```python
from build123d import *

# Parameters (mm, degrees)
ESBO_O1_R                = 6.5
RESSALTO_EXTRUS_O1_DEPTH = 15
ESBO_O4_R                = 4.5
CORTE_EXTRUS_O1_DEPTH    = 3.1
ESBO_O5_R                = 3.25
CORTE_EXTRUS_O2_DEPTH    = 16.036954479
CHANFRO1_SIZE            = 0.5
FILETE1_R                = 0.5
FILETE2_R                = 0.5


with BuildPart() as part:
    # Esboço1 → Ressalto-extrusão1 (new body)
    with BuildSketch(Plane(origin=(0, 0, 0), x_dir=(1, 0, 0), z_dir=(0, 1, 0))):
        with Locations(Location((0, 0, 0), (0, 0, 270))):
            Circle(ESBO_O1_R)
    extrude(amount=RESSALTO_EXTRUS_O1_DEPTH)

    # Esboço4 → Corte-extrusão1 (cut)
    with BuildSketch(Plane.XZ):
        with Locations(Location((0, 0, 0), (0, 0, 270))):
            Circle(ESBO_O4_R)
    extrude(amount=-CORTE_EXTRUS_O1_DEPTH, mode=Mode.SUBTRACT)

    # Esboço5 → Corte-extrusão2 (cut, through all)
    with BuildSketch(Plane.XZ.offset(-3.1)):
        with Locations(Location((0, 0, 0), (0, 0, 270))):
            Circle(ESBO_O5_R)
    extrude(amount=-CORTE_EXTRUS_O2_DEPTH, mode=Mode.SUBTRACT)

    # Chanfro1
    chanfro1_edges = [part.edges().sort_by_distance(p)[0] for p in [
        (0, 0, 4.5),
    ]]
    chamfer(chanfro1_edges, length=CHANFRO1_SIZE)

    # Filete1
    filete1_edges = [part.edges().sort_by_distance(p)[0] for p in [
        (0, 3.1, 3.25),
    ]]
    fillet(filete1_edges, radius=FILETE1_R)

    # Filete2
    filete2_edges = [part.edges().sort_by_distance(p)[0] for p in [
        (0, 15, 3.25),
    ]]
    fillet(filete2_edges, radius=FILETE2_R)


solid = part.part
```
Read the model definition and answer for the solid it produces. Units are mm, in the model's axes. A direction names the side the tool comes from. Round coordinates to 2 decimals unless told otherwise and drop trailing zeros. Write each loop counter-clockwise with the first axis right and the second up, starting at its lowest first coordinate (ties: lowest second). Pieces come first, ordered by that corner, then holes. Notation, with made-up numbers: (10.5, 19) - (57.5, 19) arc R20 ccw to (57.5, 54) - close; hole circle Ø1 at (78, 0). An arc over 180 degrees is marked (long way). One line per item, written item: value.
Q1. Find section A-A (x = 0). Determine the outline of the cut face in (y, z), and give its area (3 significant figures).
The answers:
outline: (0, -6.5) - (15, -6.5) - (15, -3.75) arc R0.5 ccw to (14.5, -3.25) - (3.6, -3.25) arc R0.5 ccw to (3.1, -3.75) - (3.1, -4.5) - (0.5, -4.5) - (0, -5) - close; (0, 5) - (0.5, 4.5) - (3.1, 4.5) - (3.1, 3.75) arc R0.5 ccw to (3.6, 3.25) - (14.5, 3.25) arc R0.5 ccw to (15, 3.75) - (15, 6.5) - (0, 6.5) - close
area: 89.3 mm2
Q2. For a pull along Z with two mould halves and no side action, classify faces 1 (the cylindrical face through (-3.955, 7.395, -5.158)), 2 (the flat face through (-3, 15, 3)), 3 (the flat face through (4, 3.1, 1)) as pulls with the +Z half, pulls with the -Z half, needs draft (parallel to the pull), parting line crosses it, or undercut.
The answers:
face 1: parting line crosses it
face 2: needs draft
face 3: undercut
Q3. Straight lines are drawn through the part: line 1 (X direction, y = 8, z = 0); line 2 (X direction, y = 2, z = 0); line 3 (Z direction, x = 1, y = 13). For each, find the intervals that lie inside material, in ascending order. Write a range as from..to.
The answers:
line 1: x = -6.5..-3.25, 3.25..6.5
line 2: x = -6.5..-4.5, 4.5..6.5
line 3: z = -6.42..-3.09, 3.09..6.42
Q4. Find section B-B (z = 0). Determine the outline of the cut face in (x, y).
The answers:
outline: (-6.5, 0) - (-5, 0) - (-4.5, 0.5) - (-4.5, 3.1) - (-3.75, 3.1) arc R0.5 ccw to (-3.25, 3.6) - (-3.25, 14.5) arc R0.5 ccw to (-3.75, 15) - (-6.5, 15) - close; (3.25, 3.6) arc R0.5 ccw to (3.75, 3.1) - (4.5, 3.1) - (4.5, 0.5) - (5, 0) - (6.5, 0) - (6.5, 15) - (3.75, 15) arc R0.5 ccw to (3.25, 14.5) - close
Q5. Each of these flat-tipped pins is pushed along its axis until it touches: P1, Ø2.5, axis at x = 1, z = 1, coming from the -Y side; P2, Ø3, axis at y = 13.5, z = -4.5, coming from the +X side; P3, Ø1, axis at x = -5, y = 3, coming from the +Z side; P4, Ø1.5, axis at x = 3, y = 3.5, coming from the +Z side. Where does it stop, or does it pass through?
The answers:
P1: passes through
P2: stops at x = 5.77
P3: stops at z = 4.69
P4: stops at z = 6.1
Q6. Which of the six approach directions +Z, -Z, +X, -X, +Y, -Y give full straight-line access (tool end or side, diameter ignored) to faces 4 (the cylindrical face through (-1.978, 8.974, 2.579)), 5 (the cylindrical face through (1.352, 1.782, -4.292))?
The answers:
face 4: +Y, -Y
face 5: -Y
Q7. Find section C-C (y = 12). Determine the outline of the cut face in (x, z).
The answers:
outline: circle Ø13 at (0, 0); hole circle Ø6.5 at (0, 0)
Q8. Find section D-D (y = 2.5). Determine the outline of the cut face in (x, z).
The answers:
outline: circle Ø13 at (0, 0); hole circle Ø9 at (0, 0)
